For this review, take the finished solid that the model builds, in its own axes (mm). A direction names the side the tool comes from. Give positions to 0.01 mm unless a question says otherwise; leave off trailing zeros. Loops run counter-clockwise (first coordinate to the right, second up) from the corner with the lowest first, then second, coordinate; pieces in that order, holes last.
```python
from build123d import *
from build123d.topology import SkipClean

# Parameters (mm, degrees)
EXTRUDE_1_DEPTH = 0.5
EXTRUDE_2_DEPTH = 6.4
EXTRUDE_3_DEPTH = 0.5
EXTRUDE_4_DEPTH = 6.4
EXTRUDE_5_DEPTH = 0.5
EXTRUDE_START   = -7.4
EXTRUDE_6_DEPTH = 7.4


with BuildPart() as part:
    # 草图1 → 凸台-拉伸1 (new body)
    with BuildSketch(Plane(origin=(0, 0, 0), x_dir=(1, 0, 0), z_dir=(0, 1, 0))):
        with BuildLine():
            Line((11.456239028, 1.002291042), (10.46004433, 0.915135299))
            ThreePointArc((10.46004433, 0.915135299), (-10.5, 0), (10.46004433, -0.915135299))
            Line((10.46004433, -0.915135299), (11.456239028, -1.002291042))
            ThreePointArc((11.456239028, -1.002291042), (5.310109052, -10.200624582), (-5.75, -9.959292144))
            Line((-5.75, -9.959292144), (-7.25, -12.557368355))
            ThreePointArc((-7.25, -12.557368355), (-8.827040721, -11.503623434), (-10.253048327, -10.253048327))
            Line((-10.253048327, -10.253048327), (-8.131727984, -8.131727984))
            ThreePointArc((-8.131727984, -8.131727984), (-10.422539551, -4.86011001), (-11.456239028, -1.002291042))
            Line((-11.456239028, -1.002291042), (-13.448628424, -1.176602527))
            ThreePointArc((-13.448628424, -1.176602527), (-13.5, 0), (-13.448628424, 1.176602527))
            Line((-13.448628424, 1.176602527), (-11.456239028, 1.002291042))
            ThreePointArc((-11.456239028, 1.002291042), (-10.422539551, 4.86011001), (-8.131727984, 8.131727984))
            Line((-8.131727984, 8.131727984), (-10.253048327, 10.253048327))
            ThreePointArc((-10.253048327, 10.253048327), (-8.827040721, 11.503623434), (-7.25, 12.557368355))
            Line((-7.25, 12.557368355), (-5.75, 9.959292144))
            ThreePointArc((-5.75, 9.959292144), (5.310109052, 10.200624582), (11.456239028, 1.002291042))
        make_face()
    extrude(amount=EXTRUDE_1_DEPTH)

    # 草图10 → 凸台-拉伸2 (add)
    with BuildSketch(Plane(origin=(0, 0.5, 0), x_dir=(1, 0, 0), z_dir=(0, 1, 0))):
        with BuildLine():
            Line((10.46004433, -0.915135299), (11.456239028, -1.002291042))
            ThreePointArc((11.456239028, -1.002291042), (10.200624582, -5.310109052), (7.392057511, -8.809511096))
            Line((7.392057511, -8.809511096), (6.749269902, -8.043466653))
            ThreePointArc((6.749269902, -8.043466653), (9.313613748, -4.848360439), (10.46004433, -0.915135299))
        make_face()
        with BuildLine():
            Line((10.46004433, 0.915135299), (11.456239028, 1.002291042))
            ThreePointArc((11.456239028, 1.002291042), (10.187396942, 5.335442206), (7.348181349, 8.846142146))
            Line((7.348181349, 8.846142146), (6.709209057, 8.076912394))
            ThreePointArc((6.709209057, 8.076912394), (9.301536339, 4.87149071), (10.46004433, 0.915135299))
        make_face()
        with BuildLine():
            Line((6.601509895, -9.416478488), (5.991894646, -8.622482157))
            ThreePointArc((5.991894646, -8.622482157), (-10.499966218, -0.026634823), (5.94807324, 8.652769772))
            Line((5.94807324, 8.652769772), (6.553696854, 9.449817858))
            ThreePointArc((6.553696854, 9.449817858), (-11.49996307, -0.02914447), (6.601509895, -9.416478488))
        make_face()
    extrude(amount=EXTRUDE_2_DEPTH)

    # 草图11 → 凸台-拉伸3 (add)
    with BuildSketch(Plane(origin=(0, 6.9, 0), x_dir=(1, 0, 0), z_dir=(0, 1, 0))):
        with BuildLine():
            Line((10.46004433, 0.915135299), (11.456239028, 1.002291042))
            ThreePointArc((11.456239028, 1.002291042), (-11.5, 0), (11.456239028, -1.002291042))
            Line((11.456239028, -1.002291042), (10.46004433, -0.915135299))
            ThreePointArc((10.46004433, -0.915135299), (-10.5, 0), (10.46004433, 0.915135299))
        make_face()
    extrude(amount=EXTRUDE_3_DEPTH)

    # 草图12 → 凸台-拉伸4 (add)
    with BuildSketch(Plane(origin=(0, 0.5, 0), x_dir=(1, 0, 0), z_dir=(0, 1, 0))):
        with BuildLine():
            Line((-8.131727984, -8.131727984), (-8.838834765, -8.838834765))
            ThreePointArc((-8.838834765, -8.838834765), (-7.609517863, -9.916916754), (-6.25, -10.825317547))
            Line((-6.25, -10.825317547), (-5.75, -9.959292144))
            ThreePointArc((-5.75, -9.959292144), (-7.000756434, -9.123563413), (-8.131727984, -8.131727984))
        make_face()
        with BuildLine():
            Line((-10.253048327, -10.253048327), (-9.687362902, -9.687362902))
            ThreePointArc((-9.687362902, -9.687362902), (-8.340031577, -10.868940762), (-6.85, -11.864548032))
            Line((-6.85, -11.864548032), (-7.25, -12.557368355))
            ThreePointArc((-7.25, -12.557368355), (-8.827040721, -11.503623434), (-10.253048327, -10.253048327))
        make_face()
        with BuildLine():
            Line((-10.253048327, 10.253048327), (-9.687362902, 9.687362902))
            ThreePointArc((-9.687362902, 9.687362902), (-8.340031577, 10.868940762), (-6.85, 11.864548032))
            Line((-6.85, 11.864548032), (-7.25, 12.557368355))
            ThreePointArc((-7.25, 12.557368355), (-8.827040721, 11.503623434), (-10.253048327, 10.253048327))
        make_face()
        with BuildLine():
            Line((-5.75, 9.959292144), (-6.25, 10.825317547))
            ThreePointArc((-6.25, 10.825317547), (-7.609517863, 9.916916754), (-8.838834765, 8.838834765))
            Line((-8.838834765, 8.838834765), (-8.131727984, 8.131727984))
            ThreePointArc((-8.131727984, 8.131727984), (-7.000756434, 9.123563413), (-5.75, 9.959292144))
        make_face()
        with BuildLine():
            Line((-13.448628424, 1.176602527), (-12.452433726, 1.089446784))
            ThreePointArc((-12.452433726, 1.089446784), (-12.5, 0), (-12.452433726, -1.089446784))
            Line((-12.452433726, -1.089446784), (-13.448628424, -1.176602527))
            ThreePointArc((-13.448628424, -1.176602527), (-13.5, 0), (-13.448628424, 1.176602527))
        make_face()
    extrude(amount=EXTRUDE_4_DEPTH)

    # 草图13 → 凸台-拉伸5 (add)
    with BuildSketch(Plane(origin=(0, 6.9, 0), x_dir=(1, 0, 0), z_dir=(0, 1, 0))):
        with BuildLine():
            Line((-8.131727984, -8.131727984), (-10.253048327, -10.253048327))
            ThreePointArc((-10.253048327, -10.253048327), (-8.827040721, -11.503623434), (-7.25, -12.557368355))
            Line((-7.25, -12.557368355), (-5.75, -9.959292144))
            ThreePointArc((-5.75, -9.959292144), (-7.000756434, -9.123563413), (-8.131727984, -8.131727984))
        make_face()
        with BuildLine():
            Line((-7.25, 12.557368355), (-5.75, 9.959292144))
            ThreePointArc((-5.75, 9.959292144), (-7.000756434, 9.123563413), (-8.131727984, 8.131727984))
            Line((-8.131727984, 8.131727984), (-10.253048327, 10.253048327))
            ThreePointArc((-10.253048327, 10.253048327), (-8.827040721, 11.503623434), (-7.25, 12.557368355))
        make_face()
        with BuildLine():
            Line((-13.448628424, 1.176602527), (-11.456239028, 1.002291042))
            ThreePointArc((-11.456239028, 1.002291042), (-11.5, 0), (-11.456239028, -1.002291042))
            Line((-11.456239028, -1.002291042), (-13.448628424, -1.176602527))
            ThreePointArc((-13.448628424, -1.176602527), (-13.5, 0), (-13.448628424, 1.176602527))
        make_face()
    extrude(amount=EXTRUDE_5_DEPTH)

    # 草图14 → 凸台-拉伸6 (add)
    with SkipClean():  # the faces are left unmerged after this step: merging them gives an invalid solid
        with BuildSketch(Plane(origin=(0, 7.4, 0), x_dir=(1, 0, 0), z_dir=(0, 1, 0)).offset(EXTRUDE_START)):
            with BuildLine():
                Line((10.46004433, 0.915135299), (11.456239028, 1.002291042))
                ThreePointArc((11.456239028, 1.002291042), (11.5, 0), (11.456239028, -1.002291042))
                Line((11.456239028, -1.002291042), (10.46004433, -0.915135299))
                ThreePointArc((10.46004433, -0.915135299), (10.5, 0), (10.46004433, 0.915135299))
            make_face()
        extrude(amount=EXTRUDE_6_DEPTH)


solid = part.part
```
Q1. Consider section D-D on z = 5. Give the boundary of the cut face in (x, y), plus the area to 3 significant figures.
Answers:
outline: (-10.36, 0) - (-9.23, 0) - (-9.23, 7.4) - (-10.36, 7.4) - close; (9.23, 0) - (10.36, 0) - (10.36, 7.4) - (9.23, 7.4) - close
area: 16.6 mm2
Q2. For pin 1 Ø1.5 at (x, z) = (-3.5, -8) entering from -Y; pin 2 Ø1.5 at (x, z) = (6.5, 8.5) entering from -Y; pin 3 Ø3 at (x, y) = (-4.5, 6.5) entering from -Z; pin 4 Ø2 at (x, y) = (-2, 5.5) entering from -Z, all flat-tipped, find the tip position at first contact; note any pin that passes through.
Answers:
pin 1: passes through
pin 2: stops at y = 0
pin 3: stops at z = -11.1
pin 4: stops at z = -11.46
Q3. Consider section B-B on z = 0. Give the boundary of the cut face in (x, y), plus the area to 3 significant figures.
Answers:
outline: (-13.5, 0) - (-10.5, 0) - (-10.5, 7.4) - (-13.5, 7.4) - close; (10.5, 0) - (11.5, 0) - (11.5, 7.4) - (10.5, 7.4) - close; hole (-12.5, 0.5) - (-11.5, 0.5) - (-11.5, 6.9) - (-12.5, 6.9) - close
area: 23.2 mm2
Q4. For probe 1 along X at (y, z) = (7.3, 0); probe 2 along Z at (x, y) = (0, 4.5); probe 3 along X at (y, z) = (5.25, -0.5), list the stretches that pass through material, from the lowest coordinate up.
Answers:
probe 1: x = -13.5 to -10.5, 10.5 to 11.5
probe 2: z = -11.5 to -10.5, 10.5 to 11.5
probe 3: x = -13.49 to -12.49, -11.49 to -10.49, 10.49 to 11.49
Q5. Machinability: for faces 5 (the cylindrical face through (-8.848, 3.648, -11.487)), 6 (the flat face through (-8.7, 3.6, -8.7)), 7 (the cylindrical face through (-8.36, 3.655, -10.854)), which of the approach directions +Z, -Z, +X, -X, +Y, -Y give a long, thin tool a straight path to every point of the face, cutting with its end or side? Answer none if there is none.
Answers:
face 5: -Z, -X, +Y, -Y
face 6: -X, +Y, -Y
face 7: none
Q6. Mouldability with a two-part tool opening along Z and no side actions: class faces 1 (the cylindrical face through (-13.5, 3.6, 0)), 2 (the flat face through (-9, 7.4, -6)), 3 (the flat face through (6.6, 6.9, -8.8)), 4 (the flat face through (-8, 0.5, -10)) as +Z half, -Z half, draft (parallel to the pull), parting line (faces both ways), or undercut.
Answers:
face 1: parting line
face 2: draft
face 3: undercut
face 4: undercut
Q7. Consider section A-A on x = 0. Give the boundary of the cut face in (y, z).
Answers:
outline: (0, -11.5) - (7.4, -11.5) - (7.4, -10.5) - (0, -10.5) - close; (0, 10.5) - (7.4, 10.5) - (7.4, 11.5) - (0, 11.5) - close
Q8. Consider section C-C on y = 4.25. Give the boundary of the cut face in (x, z).
Answers:
outline: (-13.45, -1.18) - (-12.45, -1.09) arc R12.5 cw to (-12.45, 1.09) - (-13.45, 1.18) arc R13.5 ccw to start; (-10.25, -10.25) arc R14.5 ccw to (-7.25, -12.56) - (-6.85, -11.86) arc R13.7 cw to (-9.69, -9.69) - close; (-10.25, 10.25) - (-9.69, 9.69) arc R13.7 cw to (-6.85, 11.86) - (-7.25, 12.56) arc R14.5 ccw to start; (-8.84, -8.84) arc R12.5 ccw to (-6.25, -10.83) - (-5.75, -9.96) arc R11.5 ccw to (6.55, -9.45) - (5.95, -8.65) arc R10.5 cw (long way) to (5.99, 8.62) - (6.6, 9.42) arc R11.5 ccw to (-5.75, 9.96) - (-6.25, 10.83) arc R12.5 ccw to (-8.84, 8.84) - (-8.13, 8.13) arc R11.5 ccw to (-8.13, -8.13) - close; (6.71, -8.08) - (7.35, -8.85) arc R11.5 ccw to (7.39, 8.81) - (6.75, 8.04) arc R10.5 cw to start
